Autodesk Inventor part; units mm, degrees
ref_plane "YZ Plane" through (0, 0, 0) normal (1, 0, 0) x (0, 1, 0)
ref_plane "XZ Plane" through (0, 0, 0) normal (0, 1, 0) x (-1, 0, 0)
ref_plane "XY Plane" through (0, 0, 0) normal (0, 0, 1) x (1, 0, 0)
sketch "Skizze1" plane through (0, 0, 0) normal (0, 0, 1) x (1, 0, 0)
  line L0 (-70, 152.5) -> (70, 152.5)
  line L1 (70, 152.5) -> (70, -152.5)
  line L2 (70, -152.5) -> (-70, -152.5)
  line L3 (-70, -152.5) -> (-70, 152.5)
  line L4 (-70, 152.5) -> (70, -152.5) construction
  line L5 (70, 152.5) -> (-70, -152.5) construction
  point P0 (0, 0)
  dimension "d2" = 140
  dimension "d3" = 305
extrude "Extrusion1" add sketch "Skizze1" along normal blind 10
sketch "Skizze2" plane through (0, 0, 0) normal (0, 0, -1) x (-1, 0, 0)
  point P0 (0, 0)
  point P1 (-35, 147.5)
  dimension "d6" = 147.5
  dimension "d7" = 35
sketch "Skizze4" plane through (0, 0, 10) normal (0, 0, 1) x (1, 0, 0)
  spline S0 degree 3 poles (4.1682, 35.1897) (1.1905, 36.4598) (-2.2497, 35.1642) (-6.2549, 34.1582) (-11.736, 32.1479) (-17.2675, 27.437) (-17.3979, 22.2805) (-19.1794, 11.8373) (-24.2043, -4.2198) (-21.9122, -21.3618) (-15.7263, -32.1361) (-8.9601, -34.8731) (-7.7344, -35.2068) knots 0 0 0 0 0.027675 0.038264 0.105891 0.147773 0.191482 0.216461 0.377442 0.40617 0.483619 0.5 0.5 0.5 0.5
  spline S1 degree 3 poles (-7.7344, -35.2068) (-2.4391, -36.6482) (4.9342, -35.145) (14.3889, -31.3641) (20.2206, -28.2766) (23.0847, -23.1792) (23.281, -18.9959) (17.3062, -16.4997) (13.7398, -19.2937) (6.9074, -22.9332) (-1.1986, -27.1621) (-10.3055, -22.9326) (-14.0352, -10.4002) (-9.4599, -0.926) (-6.8333, 0.3153) (-5.9182, 2.0588) (-5.9367, 4.1791) (-8.2887, 5.2306) (-8.3641, 10.4373) (-1.0106, 14.1251) (4.0821, 20.0507) (3.0635, 26.3026) (2.9493, 28.6136) (3.7888, 29.834) (5.5778, 31.0924) (6.6132, 32.7745) (5.2458, 34.7086) (4.2657, 35.1481) (4.1682, 35.1897) knots 0.5 0.5 0.5 0.5 0.570765 0.585175 0.622993 0.62946 0.645114 0.663132 0.686116 0.69449 0.741048 0.754128 0.812208 0.823709 0.857637 0.863035 0.873446 0.900861 0.905942 0.924257 0.958178 0.971687 0.974109 0.98148 0.983255 0.99094 0.999094 1 1 1 1
  arc A0 (-7.9107, 24.207) -> (-7.9109, 20.407) centre (-6.0635, 22.307) ccw
  line L0 (-7.9107, 24.207) -> (-4.2161, 24.2069)
  arc A1 (-4.2163, 20.4069) -> (-4.2161, 24.2069) centre (-6.0635, 22.307) ccw
  line L1 (-4.2163, 20.4069) -> (-7.9109, 20.407)
  spline S2 degree 3 poles (4.1682, 35.1897) (1.1905, 36.4598) (-2.2497, 35.1642) (-6.255, 34.1582) (-11.7361, 32.1479) (-17.2675, 27.437) (-17.3979, 22.2805) (-19.1794, 11.8373) (-24.2043, -4.2198) (-21.9122, -21.3619) (-15.7263, -32.1361) (-8.9601, -34.8731) (-7.7344, -35.2068) knots 0 0 0 0 0.027675 0.038264 0.105891 0.147773 0.191482 0.216461 0.377442 0.40617 0.483619 0.5 0.5 0.5 0.5
  spline S3 degree 3 poles (-7.7344, -35.2068) (-2.4391, -36.6482) (4.9342, -35.145) (14.3889, -31.3641) (20.2206, -28.2766) (23.0847, -23.1792) (23.281, -18.9959) (17.3062, -16.4997) (13.7398, -19.2937) (6.9074, -22.9332) (-1.1986, -27.1621) (-10.3055, -22.9326) (-14.0352, -10.4002) (-9.4599, -0.926) (-6.8333, 0.3153) (-5.9182, 2.0588) (-5.9367, 4.1791) (-8.2887, 5.2306) (-8.3641, 10.4373) (-1.0106, 14.1251) (4.0821, 20.0507) (3.0635, 26.3026) (2.9493, 28.6136) (3.7888, 29.834) (5.5778, 31.0924) (6.6132, 32.7745) (5.2458, 34.7086) (4.2657, 35.1481) (4.1682, 35.1897) knots 0.5 0.5 0.5 0.5 0.570765 0.585175 0.622993 0.62946 0.645114 0.663132 0.686116 0.69449 0.741048 0.754128 0.812208 0.823709 0.857637 0.863035 0.873446 0.900861 0.905942 0.924257 0.958178 0.971687 0.974109 0.98148 0.983255 0.99094 0.999094 1 1 1 1
  line L2 (-4.2163, 20.4069) -> (-7.9109, 20.407)
  arc A2 (-4.2163, 20.4069) -> (-4.2161, 24.2069) centre (-6.0635, 22.307) ccw
  line L3 (-7.9107, 24.207) -> (-4.2161, 24.2069)
  arc A3 (-7.9107, 24.207) -> (-7.9109, 20.407) centre (-6.0635, 22.307) ccw
  line L4 (-22.9949, 35.8296) -> (22.9949, 35.8296) construction
  line L5 (22.9949, 35.8296) -> (22.9949, -35.8296) construction
  line L6 (22.9949, -35.8296) -> (-22.9949, -35.8296) construction
  line L7 (-22.9949, -35.8296) -> (-22.9949, 35.8296) construction
  line L8 (-22.9949, 35.8296) -> (22.9949, -35.8296) construction
  line L9 (-22.9949, -35.8296) -> (22.9949, 35.8296) construction
  point P0 (0, 0)
  point P1 (0, 0)
  point P2 (0, 0)
hole "Bohrung2" at (35, 147.5, 0) direction (0, 0, 1) diameter 4.5 end through all counterbore diameter 8 counterbore depth 4.4
pattern_linear "Rechteckige Anordnung2" count 3 spacing 47.5 along (0, -1, 0) count 2 spacing 70 along (-1, 0, 0) of "Bohrung2"
mirror "Spiegeln2" about plane through (0, 0, 0) normal (0, 1, 0) of "Bohrung2", "Rechteckige Anordnung2"
sketch "Skizze7" plane through (0, 0, 10) normal (0, 0, 1) x (1, 0, 0)
  line L0 (-70, -152.5) -> (70, -152.5)
  line L1 (-30, 152.5) -> (30, 152.5)
  line L2 (30, 152.5) -> (30, -152.5)
  line L3 (30, -152.5) -> (-30, -152.5)
  line L4 (-30, -152.5) -> (-30, 152.5)
  line L5 (-70, 152.5) -> (-70, -152.5)
  line L6 (70, 152.5) -> (-70, 152.5)
  point P0 (0, 0)
  dimension "d99" = 60
  dimension "d100" = 40
extrude "Extrusion4" cut sketch "Skizze7" against normal blind 5 contours L4 L1 L2 L0
sketch "Skizze8" plane through (0, 0, 5) normal (0, 0, 1) x (1, 0, 0)
  arc A0 (-32.75, -100) -> (-32.75, -100) centre (-35, -100) ccw
  arc A1 (37.25, -100) -> (37.25, -100) centre (35, -100) ccw
  arc A2 (31, 100) -> (31, 100) centre (35, 100) ccw
  arc A3 (-32.75, 100) -> (-32.75, 100) centre (-35, 100) ccw
  arc A4 (37.25, 100) -> (37.25, 100) centre (35, 100) ccw
  line L0 (30, -152.5) -> (-30, -152.5)
  line L1 (30, 152.5) -> (30, -152.5)
  line L2 (-30, 152.5) -> (30, 152.5)
  line L3 (-30, -152.5) -> (-30, 152.5)
  arc A5 (31, -100) -> (31, -100) centre (35, -100) ccw construction
  arc A6 (-39, 100) -> (-39, 100) centre (-35, 100) ccw construction
  line L4 (0, -107) -> (0, -107)
  line L5 (7, -100) -> (7, 100)
  line L6 (0, 107) -> (0, 107)
  line L7 (-7, 100) -> (-7, -100)
  arc A7 (-7, -100) -> (0, -107) centre (0, -100) ccw
  arc A8 (0, -107) -> (7, -100) centre (0, -100) ccw
  arc A9 (7, 100) -> (0, 107) centre (0, 100) ccw
  arc A10 (0, 107) -> (-7, 100) centre (0, 100) ccw
  point P0 (0, 0)
  point P1 (0, 107)
  point P2 (0, -107)
  dimension "d157" = 14
  dimension "d158" = 7
  dimension "d159" = 52.5
  dimension "d160" = 200
extrude "Extrusion5" cut sketch "Skizze8" against normal through all contours A8 A7 L7 A10 A9 L5
sketch "Skizze9" plane through (0, 0, 5) normal (0, 0, 1) x (1, 0, 0)
  line L0 (30, -152.5) -> (-30, -152.5)
  point P0 (0, 0)
  point P1 (-22.5, -125.1)
  point P2 (0, -152.5)
  dimension "d116" = 22.5
  dimension "d117" = 27.4
hole "Bohrung3" at (-22.5, -125.1, 5) direction (0, 0, -1) diameter 4.134 end through all
chamfer "Fasen2" distance 0.5 angle 45 2 edges at (-22.5, -123.033, 5) (-22.5, -123.033, 0)
pattern_linear "Rechteckige Anordnung3" count 2 spacing 45 along (1, 0, 0) count 2 spacing 13 along (0, 1, 0) of "Bohrung3", "Fasen2"
sketch "Skizze10" plane through (0, 0, 10) normal (0, 0, 1) x (1, 0, 0)
  circle A0 centre (35, -147.5) radius 2.25
  circle A1 centre (-35, -52.5) radius 2.25
  circle A2 centre (-35, -100) radius 2.25
  circle A3 centre (35, -100) radius 2.25
  circle A4 centre (35, 100) radius 2.25
  circle A5 centre (35, 147.5) radius 2.25
  circle A6 centre (-35, 100) radius 2.25
  circle A7 centre (-35, 52.5) radius 2.25
  point P0 (0, 0)
  point P1 (35, -123.75)
  point P2 (-35, -76.25)
  point P3 (-35, 123.75)
  point P4 (35, 76.25)
  dimension "d137" = 23.75
  dimension "d138" = 23.75
  dimension "d149" = 23.75
  dimension "d150" = 23.75
hole "Bohrung4" at (35, -123.75, 10) at (-35, -76.25, 10) at (-35, 123.75, 10) at (35, 76.25, 10) direction (0, 0, -1) diameter 4 depth 5.5 countersink diameter 5 countersink angle 90
chamfer "Fasen3" distance 1 angle 45 4 edges at (-7, 0, 5) (0, 107, 5) (7, 0, 5) (0, -107, 5)
equation "\"d2\" = Breite_aussen + 2 * Montierflaeche"
equation "\"d3\" = 2 * Laenge_aussen + Zwischenteil"
equation "\"d4\" = Wanddicke"
equation "\"d95\" = -0.5 * Wanddicke + 0.5 * Laenge_aussen"
equation "\"d98\" = Breite_aussen - Wanddicke"
equation "\"d99\" = Breite_aussen - 2 * Wanddicke"
equation "\"d100\" = Wanddicke + Montierflaeche"
equation "\"d101\" = Absatz"
equation "\"Breite_aussen\" = 80"
equation "\"Laenge_aussen\" = 105"
equation "\"Wanddicke\" = 10"
equation "\"Laenge_innen\" = Laenge_aussen - Wanddicke"
equation "\"Absatz\" = 5"
equation "\"Kolbenanbindung_Breite\" = 14"
equation "\"d135\" = 0.5 * d134"
properties part number "TS_V1_Fallmagazin_Boden_int"
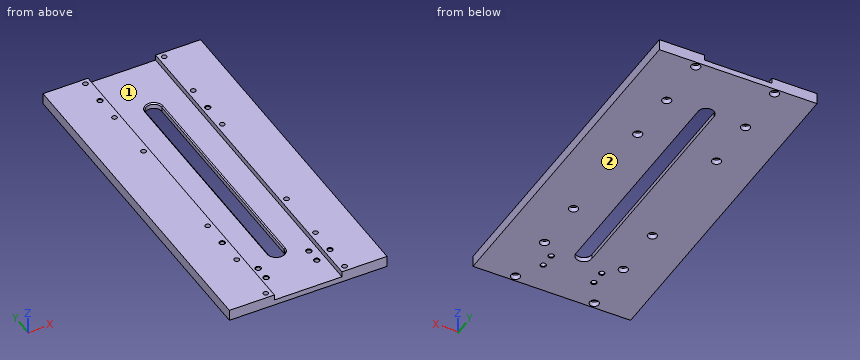
Source: CAD feature listing. Evaluate the final solid. Frame: model axes, mm. Face numbers are marked on the shaded views. Coordinates: 2 decimals unless noted, no trailing zeros. Loops run counter-clockwise (first coordinate to the right, second up) from the corner with the lowest first, then second, coordinate; pieces in that order, holes last. Notation, with made-up numbers: M 7,74.5 L 25,74.5 A17 cw 25,107.5 Z; hole C -35.75,-12.5 d4. An arc over 180 degrees is marked long. Use a Markdown table: item, result. Add a question column.
Q1. Material intervals for L1, parallel to X at y = 100, z = 7.5; L2, parallel to X at y = -112.1, z = 1.35; L3, parallel to X at y = -100, z = 3.05, sorted ascending.
Q2. Section query A-A, the plane y = -21. Return loops of the section in (x, z).
Q3. Draft query along X for the marked faces 1 and 2. Return one class per face: pulls with the +X half, pulls with the -X half, needs draft (parallel to the pull), parting line crosses it, or undercut.
Q4. First-contact query: pin 1 (10 mm diameter, centred on x = 24.5, y = -27.5, fed in from +Z); pin 2 (7 mm diameter, centred on x = -35, y = -52.5, fed in from -Z); pin 3 (4.5 mm diameter, centred on x = -35, y = -76.25, fed in from +Z). Flat tips, straight axial feed; report the tip coordinate or a pass-through.
Result:
| question | item | result |
|---|---|---|
| 1 | L1 | x = -70 to -37.25, -32.75 to -30, 30 to 32.75, 37.25 to 70 |
| 1 | L2 | x = -70 to -24.57, -20.43 to 20.43, 24.57 to 70 |
| 1 | L3 | x = -70 to -39, -31 to -7, 7 to 31, 39 to 70 |
| 2 | outline | M -70,0 L -7,0 L -7,4 L -8,5 L -30,5 L -30,10 L -70,10 Z; M 7,0 L 70,0 L 70,10 L 30,10 L 30,5 L 8,5 L 7,4 Z |
| 3 | face 1 | undercut |
| 3 | face 2 | needs draft |
| 4 | pin 1 | stops at z = 5 |
| 4 | pin 2 | stops at z = 4.4 |
| 4 | pin 3 | stops at z = 9.75 |
